Read the model definition and answer for the solid it produces. Units are mm, in the model's axes. A direction names the side the tool comes from. Round coordinates to 2 decimals unless told otherwise and drop trailing zeros. Write each loop counter-clockwise with the first axis right and the second up, starting at its lowest first coordinate (ties: lowest second). Pieces come first, ordered by that corner, then holes. Notation, with made-up numbers: (56, 10.25) - (95, 10.25) arc R29 cw to (95, 33.25) - close; hole circle Ø4 at (-38, -25). An arc over 180 degrees is marked (long way). Use one line per item in the form item = value. Start each with the question number.
1) Each of these flat-tipped pins is pushed along its axis until it touches: pin 1 (12 mm diameter, centred on y = 732.5, z = 21.5, fed in from -X); pin 2 (3 mm diameter, centred on x = -733, z = 86.5, fed in from -Y); pin 3 (5 mm diameter, centred on x = -649, z = 115.5, fed in from -Y) (3 decimals). Where does it stop, or does it pass through?
2) Consider line 1 along Y through (x, z) = (-430, 68); line 2 along Y through (x, z) = (-286, 158.5); line 3 along X through (y, z) = (307, 127). Determine where each line is inside the solid, lowest interval first. Write a range as from..to.
3) The part is cut by section A-A, the plane x = -672. Give the vertices of the cut face in (y, z), plus the area to 3 significant figures.
4) The part is cut by section C-C, the plane y = 550. Give the vertices of the cut face in (x, z), plus the area to 3 significant figures.
5) For a pull along X with two mould halves and no side action, classify faces 4 (the face through (-530.979, 248.555, 101.4)), 5 (the face through (-615.742, 925.036, 101.4)), 6 (the face through (-156, 487, 200)) as released by +X, released by -X, zero draft, split by the parting line, or undercut.
6) For faces 1 (the face through (-398, 240, 99)), 2 (the face through (-387, 910, 99)), 3 (the face through (-241.05, 690.04, 101.4)), determine the directions among +Z, -Z, +X, -X, +Y, -Y from which every point of the face is accessible in a straight line to the end or side of a thin tool.
7) The part is cut by section D-D, the plane x = -564. Give the vertices of the cut face in (y, z), plus the area to 3 significant figures.
from build123d import *

# Parameters (mm, degrees)
RESSALTO_EXTRUS_O1_DEPTH = 200
FILETE1_R                = 200
FILETE2_R                = 200
FILETE3_R                = 70
FILETE4_R                = 70
FILETE5_R                = 30
FILETE6_R                = 50
FILETE7_R                = 50
FILETE8_R                = 150


with BuildPart() as part:
    # Esboço1 → Ressalto-extrusão1 (new body)
    with BuildSketch(Plane.XY):
        Polygon((0, 0), (0, 910), (-630, 910), (-630, 960), (-850, 960), (-850, 710), (-220, 710), (-220, 240), (-540, 240), (-540, 270), (-900, 270), (-900, 210), (-540, 0), align=None)
    extrude(amount=RESSALTO_EXTRUS_O1_DEPTH)

    # Filete1
    filete1_edges = [part.edges().sort_by_distance(p)[0] for p in [
        (0, 910, 100),
    ]]
    fillet(filete1_edges, radius=FILETE1_R)

    # Filete2
    filete2_edges = [part.edges().sort_by_distance(p)[0] for p in [
        (0, 0, 100),
    ]]
    fillet(filete2_edges, radius=FILETE2_R)

    # Filete3
    filete3_edges = [part.edges().sort_by_distance(p)[0] for p in [
        (-220, 710, 100),
    ]]
    fillet(filete3_edges, radius=FILETE3_R)

    # Filete4
    filete4_edges = [part.edges().sort_by_distance(p)[0] for p in [
        (-220, 240, 100),
    ]]
    fillet(filete4_edges, radius=FILETE4_R)

    # Filete5
    filete5_edges = [part.edges().sort_by_distance(p)[0] for p in [
        (-540, 240, 100),
    ]]
    fillet(filete5_edges, radius=FILETE5_R - 0.0001)  # a hair under: the kernel refuses the full size

    # Filete6
    filete6_edges = [part.edges().sort_by_distance(p)[0] for p in [
        (-630, 910, 100),
    ]]
    fillet(filete6_edges, radius=FILETE6_R - 0.0001)  # a hair under: the kernel refuses the full size

    # Filete7
    filete7_edges = [part.edges().sort_by_distance(p)[0] for p in [
        (-900, 210, 100),
    ]]
    fillet(filete7_edges, radius=FILETE7_R)

    # Filete8
    filete8_edges = [part.edges().sort_by_distance(p)[0] for p in [
        (-540, 0, 100),
    ]]
    fillet(filete8_edges, radius=FILETE8_R)


solid = part.part
Geometry results:
q1.pin_1 = -850
q1.pin_2 = 111.71
q1.pin_3 = 62.125
q2.line_1 = 0..240, 710..910
q2.line_2 = 0..240.11, 709.89..910
q2.line_3 = -220.06..0
q3.outline = (77, 0) - (270, 0) - (270, 200) - (77, 200) - close; (710, 0) - (960, 0) - (960, 200) - (710, 200) - close
q3.area = 88,600 mm2
q4.outline = (-220, 0) - (0, 0) - (0, 200) - (-220, 200) - close
q4.area = 44,000 mm2
q5.face_4 = undercut
q5.face_5 = released by +X
q5.face_6 = zero draft
q6.face_1 = +Z, -Z
q6.face_2 = +Z, -Z, +X, +Y
q6.face_3 = +Z, -Z, -X
q7.outline = (14.6, 0) - (270, 0) - (270, 200) - (14.6, 200) - close; (710, 0) - (910, 0) - (910, 200) - (710, 200) - close
q7.area = 91,100 mm2
